from build123d import *

# Parameters (mm, degrees)
BOSS_EXTRU_1_DEPTH      = 10
ESQUISSE3_R             = 2.05
ESQUISSE3_R_2           = 2.1
ENL_V_MAT_EXTRU_1_DEPTH = 56.474274361
CONG_1_R                = 5


with BuildPart() as part:
    # Esquisse1 → Boss.-Extru.1 (new body)
    with BuildSketch(Plane.XY):
        Polygon((16.90473047, -36.252311481), (26.618508055, -31.722702604), (38.913655488, -14.163412304), (40.781920359, 7.190952884), (31.722702604, 26.618508055), (-26.618508055, 31.722702604), (-38.913655488, 14.163412304), (-40.781920359, -7.190952884), (-31.722702604, -26.618508055), (-22.943057454, -32.766081772), align=None)
    extrude(amount=BOSS_EXTRU_1_DEPTH)

    # Esquisse3 → Enlèv. mat.-Extru.1 (cut, through all)
    with BuildSketch(Plane(origin=(0, 0, 0), x_dir=(-1, 0, 0), z_dir=(0, 0, -1))):
        with Locations((-26.618508055, 22.705871893)):
            Circle(ESQUISSE3_R)
        with Locations((22.943057454, 26.554275329)):
            Circle(ESQUISSE3_R)
        with Locations((29.737818366, 18.469938184)):
            Circle(ESQUISSE3_R_2)
        with Locations((34.806654387, 3.73808347)):
            Circle(ESQUISSE3_R)
        with Locations((32.981605632, -11.73414452)):
            Circle(ESQUISSE3_R_2)
        with Locations((22.943057454, -28.537832938)):
            Circle(ESQUISSE3_R_2)
        with Locations((-18.601253659, -30.822032576)):
            Circle(ESQUISSE3_R_2)
        with Locations((-29.737818366, -18.469938184)):
            Circle(ESQUISSE3_R_2)
        with Locations((-34.806654387, -3.73808347)):
            Circle(ESQUISSE3_R)
        with Locations((-32.981605632, 11.73414452)):
            Circle(ESQUISSE3_R_2)
    extrude(amount=-ENL_V_MAT_EXTRU_1_DEPTH, mode=Mode.SUBTRACT)

    # Congé1
    cong_1_edges = [part.edges().sort_by_distance(p)[0] for p in [
        (40.781920359, 7.190952884, 5),
        (38.913655488, -14.163412304, 5),
        (26.618508055, -31.722702604, 5),
        (-31.722702604, -26.618508055, 5),
        (-40.781920359, -7.190952884, 5),
        (-38.913655488, 14.163412304, 5),
    ]]
    fillet(cong_1_edges, radius=CONG_1_R)


solid = part.part
Design review of the part built by this model. Coordinates are the model's own, in mm. Coordinates: 2 decimals unless noted, no trailing zeros. Order: outer loops, then holes, each group sorted by start corner. A loop starts at its lowest first (then second) coordinate and runs counter-clockwise, first axis right, second up. Notation, with made-up numbers: (-38, 2) -> (17, 2) arc R29 ccw to (17, 25) -> close; hole circle Ø2 at (45.25, 36.5). An arc over 180 degrees is marked (long way). One line per item, written item: value.
1) We need section C-C, the plane y = -7.5. Give the boundary of the cut face in (x, z).
Output values:
outline: (-40.54, 0) -> (39.5, 0) -> (39.5, 10) -> (-40.54, 10) -> close
2) We need section A-A, the plane z = 8. Count the separate pieces of the cut face and the enclosed holes in it, then the cut area to 3 significant figures.
Output values:
separate pieces: 1
enclosed holes: 10
area: 4,410 mm2
3) We need section B-B, the plane x = 13. Give the boundary of the cut face in (y, z).
Output values:
outline: (-35.91, 0) -> (28.26, 0) -> (28.26, 10) -> (-35.91, 10) -> close
4) Clearance check with flat-ended pins moving along their axes: P1, Ø2, axis at x = 5, z = 5, coming from the -Y side; P2, Ø3.5, axis at x = 32.98, y = 11.73, coming from the +Z side; P3, Ø2, axis at y = 23, z = 4, coming from the +X side; P4, Ø1, axis at y = -16, z = 6, coming from the +X side. State where each tip first meets the part, or that it passes through.
Output values:
P1: stops at y = -35.3
P2: passes through
P3: stops at x = 33.88
P4: stops at x = 37.98
5) Draft analysis for pull direction X (two halves, no side actions). For faces 1 (the face through (-1, -2, 10)), 2 (the face through (17.472, -29.051, 4.93)), 3 (the face through (32.69, -23.05, 4.93)), state which applies: +X half, -X half, draft (parallel to the pull), parting line (faces both ways), or undercut.
Output values:
face 1: draft
face 2: undercut
face 3: +X half
6) To check wall thickness, follow probe 1 along Y at (x, z) = (-23, 6.5); probe 2 along Y at (x, z) = (33.5, 5.75); probe 3 along X at (y, z) = (-29.5, 4.25). State the ranges of each line that lie inside material, in increasing order. Write a range as [from, to].
Output values:
probe 1: y = [-32.73, -30.64], [-26.44, 24.51], [28.6, 31.41]
probe 2: y = [-21.89, -5.32], [-2.16, 9.7], [13.77, 22.81]
probe 3: x = [-27.61, -24.81], [-21.08, 16.97], [20.23, 28.17]
